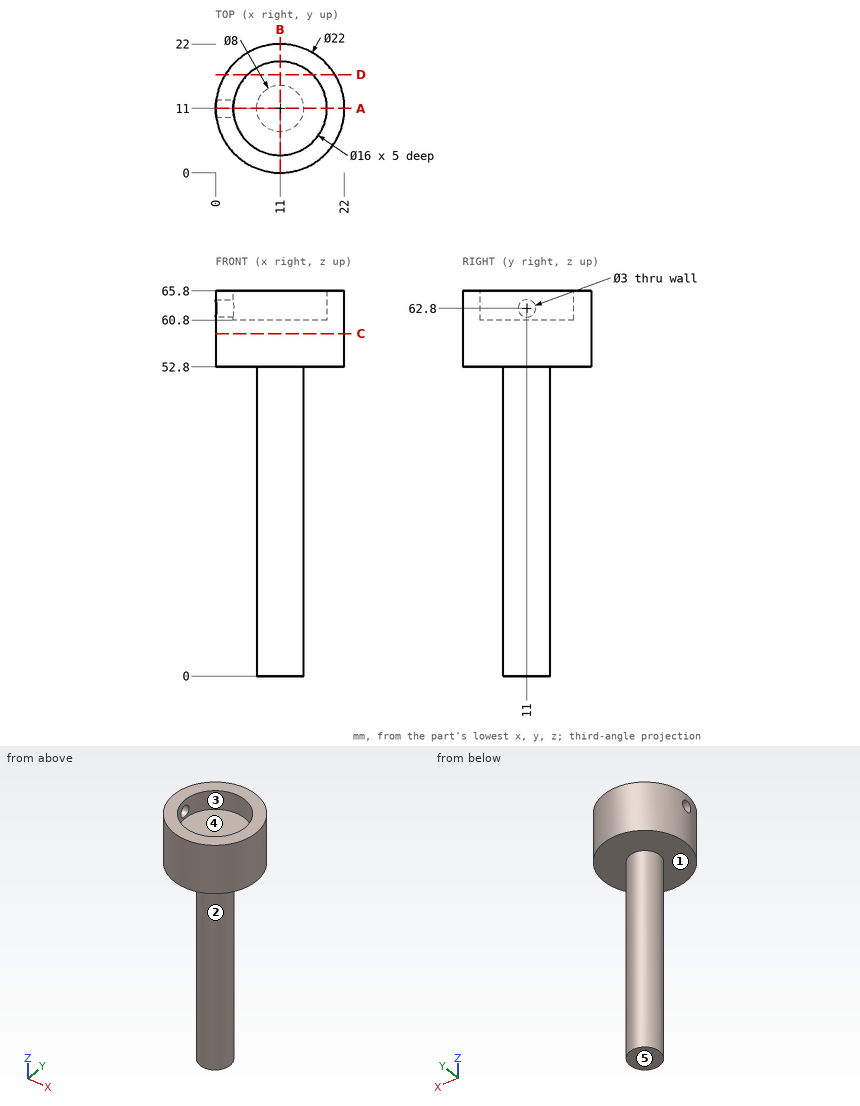
Can you work these out from the drawing? Everything is in mm from the part's minimum corner. A direction names the side the tool comes from. Round coordinates to 2 decimals unless told otherwise and drop trailing zeros. Write each loop counter-clockwise with the first axis right and the second up, starting at its lowest first coordinate (ties: lowest second). Pieces come first, ordered by that corner, then holes.
1. Suppose I cut it at D-D (y = 16.75). List the corners of the cut face in (x, z) for me, and give its area (3 significant figures).
2. I need wall thicknesses on L1, parallel to Y at x = 11, z = 62.2; L2, parallel to Z at x = 10.25, y = 2.5; L3, parallel to Z at x = 14, y = 6.25. Which ranges of each line are inside material? Lowest first, please.
3. Will these pins go through, and if not, where does the flat tip stop? pin 1 Ø8 at (y, z) = (3.5, 57.5) entering from -X; pin 2 Ø2 at (y, z) = (12.5, 23) entering from +X; pin 3 Ø3 at (x, z) = (9, 24) entering from +Y.
4. Suppose I cut it at C-C (z = 58.5). List the corners of the cut face in (x, y) for me, and give its area (3 significant figures).
5. Suppose I cut it at B-B (x = 11). List the corners of the cut face in (y, z) for me, and give its area (3 significant figures).
6. For the marked faces 4 and 5, which set-ups out of +Z, -Z, +X, -X, +Y, -Y let a thin tool reach every point of the face, with its end or its side?
7. If we mould it in two halves opening along Y, with no side actions, what happens to the marked faces 1, 2 and 3? For each: released by +Y, released by -Y, zero draft, split by the parting line, or undercut.
8. Suppose I cut it at A-A (y = 11). List the corners of the cut face in (x, z) for me.
Answer sheet:
1. outline: (1.62, 52.8) - (20.38, 52.8) - (20.38, 65.8) - (16.56, 65.8) - (16.56, 60.8) - (5.44, 60.8) - (5.44, 65.8) - (1.62, 65.8) - close
1. area: 188 mm2
2. L1: y = 0 to 3, 19 to 22
2. L2: z = 52.8 to 65.8
2. L3: z = 52.8 to 60.8
3. pin 1: stops at x = 0.57
3. pin 2: stops at x = 14.97
3. pin 3: stops at y = 14.97
4. outline: circle Ø22 at (11, 11)
4. area: 380 mm2
5. outline: (0, 52.8) - (7, 52.8) - (7, 0) - (15, 0) - (15, 52.8) - (22, 52.8) - (22, 65.8) - (19, 65.8) - (19, 60.8) - (3, 60.8) - (3, 65.8) - (0, 65.8) - close
5. area: 628 mm2
6. face 4: +Z
6. face 5: -Z, +X, -X, +Y, -Y
7. face 1: zero draft
7. face 2: split by the parting line
7. face 3: undercut
8. outline: (0, 52.8) - (7, 52.8) - (7, 0) - (15, 0) - (15, 52.8) - (22, 52.8) - (22, 65.8) - (19, 65.8) - (19, 60.8) - (3, 60.8) - (3, 61.3) - (0, 61.3) - close; (0, 64.3) - (3, 64.3) - (3, 65.8) - (0, 65.8) - close
